Design review of the part shown in the three views and the two pictorial views. Dimensions are in mm from the part's minimum x, y and z. A direction names the side the tool comes from. Round coordinates to 2 decimals unless told otherwise and drop trailing zeros. Order: outer loops, then holes, each group sorted by start corner. A loop starts at its lowest first (then second) coordinate and runs counter-clockwise, first axis right, second up. Notation, with made-up numbers: (-23.75, 60.25) -> (4.25, 60.25) arc R21 ccw to (4.25, 83.25) -> close; hole circle Ø3 at (36, 57.5). An arc over 180 degrees is marked (long way). Put each result on its own line as item: value. Start each with the question number.
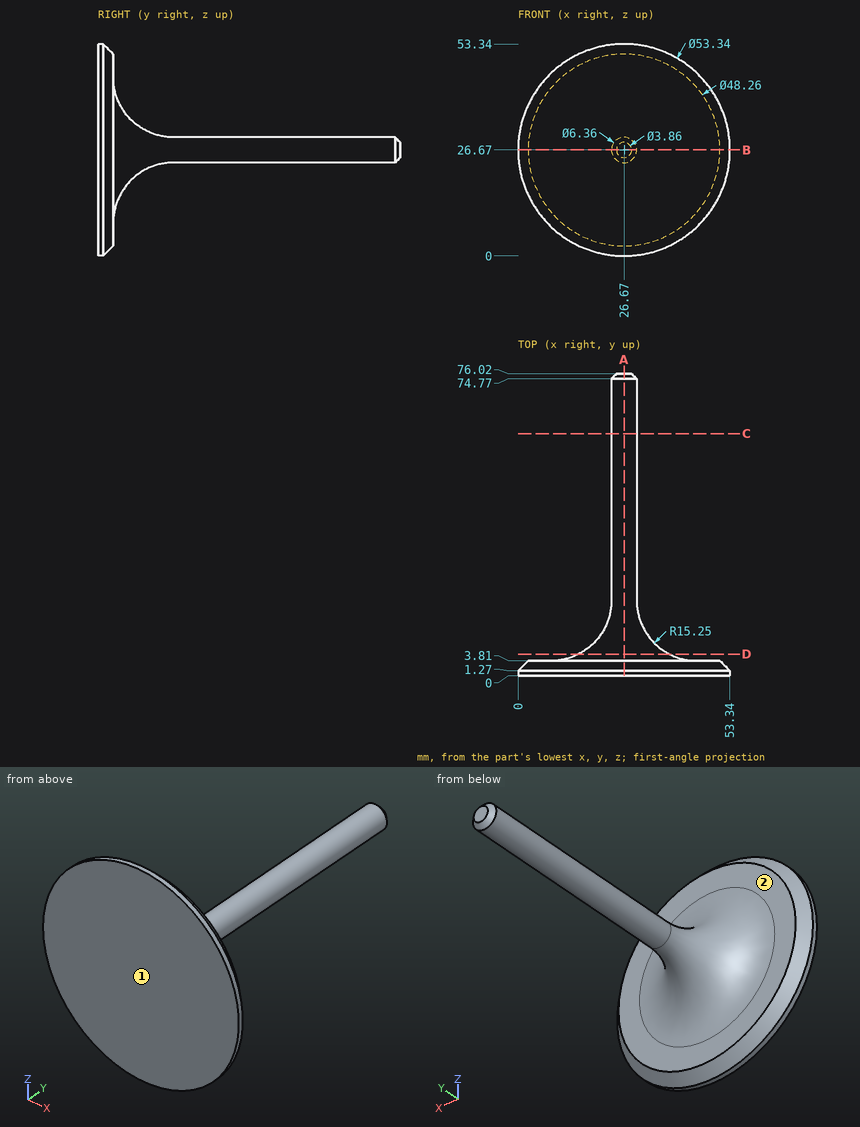
Q1. Wall thickness on probe 1 along Y at (x, z) = (30.5, 7); probe 2 along X at (y, z) = (51.5, 27); probe 3 along Z at (x, y) = (25, 20.5): over which ranges is each line inside the solid? List them lowest first. Write a range as [from, to].
Q2. Take a section at B-B on z = 26.67. Give the boundary of the cut face in (x, y).
Q3. Take a section at D-D on y = 5.5. Give the boundary of the cut face in (x, z).
Q4. Take a section at C-C on y = 61. Give the boundary of the cut face in (x, z), and give its area (3 significant figures).
Q5. Take a section at A-A on x = 26.67. Give the boundary of the cut face in (y, z), and give its area (3 significant figures).
Q6. For the marked faces 1 and 2, list the 3-axis set-ups (+Z, -Z, +X, -X, +Y, -Y) from which the entire face can be reached by the end or side of a thin tool; tool diameter is ignored.
Q7. Clearance check with flat-ended pins moving along their axes: pin 1 Ø5 at (x, y) = (33.5, 30) entering from +Z; pin 2 Ø10 at (x, y) = (27.5, 68) entering from +Z; pin 3 Ø3 at (x, z) = (22.5, 21) entering from +Y; pin 4 Ø3 at (x, z) = (8, 13.5) entering from +Y. State where each tip first meets the part, or that it passes through.
Calculated:
1. probe 1: y = [0, 3.81]
1. probe 2: x = [23.51, 29.83]
1. probe 3: z = [23.96, 29.38]
2. outline: (0, 0) -> (53.34, 0) -> (53.34, 1.27) -> (50.8, 3.81) -> (45.1, 3.81) arc R15.25 cw to (29.85, 19.06) -> (29.85, 74.77) -> (28.6, 76.02) -> (24.74, 76.02) -> (23.49, 74.77) -> (23.49, 19.06) arc R15.25 cw to (8.24, 3.81) -> (2.54, 3.81) -> (0, 1.27) -> close
3. outline: circle Ø22.9 at (26.67, 26.67)
4. outline: circle Ø6.36 at (26.67, 26.67)
4. area: 31.8 mm²
5. outline: (0, 0) -> (1.27, 0) -> (3.81, 2.54) -> (3.81, 8.24) arc R15.25 cw to (19.06, 23.49) -> (74.77, 23.49) -> (76.02, 24.74) -> (76.02, 28.6) -> (74.77, 29.85) -> (19.06, 29.85) arc R15.25 cw to (3.81, 45.1) -> (3.81, 50.8) -> (1.27, 53.34) -> (0, 53.34) -> close
5. area: 754 mm²
6. face 1: +Z, -Z, +X, -X, -Y
6. face 2: +Y
7. pin 1: passes through
7. pin 2: stops at z = 29.85
7. pin 3: stops at y = 10.91
7. pin 4: stops at y = 3.81
